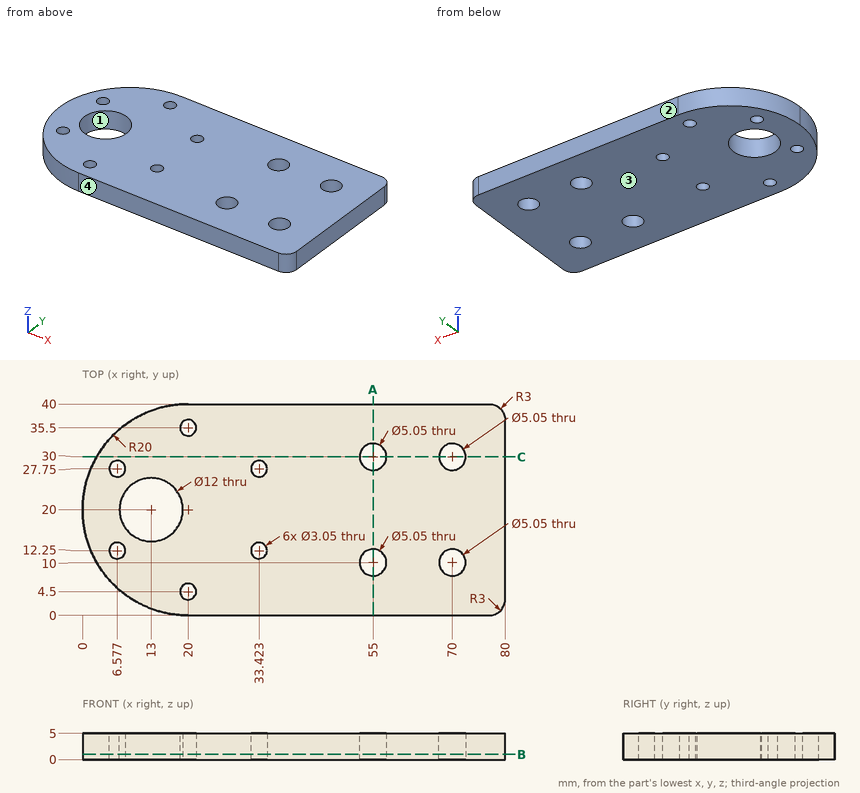
Study the drawing (mm; zero at the part's minimum x, y, z) and answer. Round coordinates to 2 decimals unless told otherwise and drop trailing zeros. Order: outer loops, then holes, each group sorted by start corner. A loop starts at its lowest first (then second) coordinate and runs counter-clockwise, first axis right, second up. Notation, with made-up numbers: (36, 24.5) - (52, 24.5) arc R21 ccw to (52, 51.5) - close; hole circle Ø5 at (89, 22). An arc over 180 degrees is marked (long way). Use one line per item in the form item = value. Start each with the question number.
(1) The part is cut by section C-C (y = 30). Give the vertices of the cut face in (x, z) (1 decimal), then the cut area to 3 significant figures.
(2) A flat-ended cylindrical pin translates along its axis: pin 1 Ø1.5 at (y, z) = (21.5, 2.5) entering from -X. Find the tip coordinate at first contact, or state that the pin passes through.
(3) The part is cut by section A-A (x = 55). Give the vertices of the cut face in (y, z) (1 decimal).
(4) Determine the mould class of the marked faces 1, 2, 3 and 4 for opening direction Y: +Y half, -Y half, draft (parallel to the pull), parting line (faces both ways), or undercut.
(5) Find the intervals of material crossed by line 1 along X through (y, z) = (30.5, 3.9) (1 decimal); line 2 along X through (y, z) = (15.5, 4.05) (1 decimal); line 3 along Y through (x, z) = (32.5, 3.3) (1 decimal), in increasing order. Write a range as from..to.
(6) The part is cut by section B-B (z = 1). Count the separate pieces of the cut face and the enclosed holes in it, then the cut area to 3 significant figures.
Checked values:
q1.outline = (2.7, 0) - (52.5, 0) - (52.5, 5) - (2.7, 5) - close; (57.5, 0) - (67.5, 0) - (67.5, 5) - (57.5, 5) - close; (72.5, 0) - (80, 0) - (80, 5) - (72.5, 5) - close
q1.area = 336 mm^2
q2.pin_1 = 0.01
q3.outline = (0, 0) - (7.5, 0) - (7.5, 5) - (0, 5) - close; (12.5, 0) - (27.5, 0) - (27.5, 5) - (12.5, 5) - close; (32.5, 0) - (40, 0) - (40, 5) - (32.5, 5) - close
q4.face_1 = undercut
q4.face_2 = +Y half
q4.face_3 = draft
q4.face_4 = -Y half
q5.line_1 = 3..52.5, 57.5..67.5, 72.5..80
q5.line_2 = 0.5..9, 17..80
q5.line_3 = 0..11, 13.5..26.5, 29..40
q6.separate_pieces = 1
q6.enclosed_holes = 11
q6.area = 2,790 mm^2
